```python
from build123d import *

# Parameters (mm, degrees)
SKETCH_R      = 6.05
SKETCH_R_2    = 2.2
PAD_DEPTH     = 6
POCKET_DEPTH  = 3.5
SKETCH002_R   = 8.05
SKETCH002_R_2 = 6.05
PAD001_DEPTH  = 4
CHAMFER_SIZE  = 0.5


with BuildPart() as part:
    # Sketch → Pad (new body)
    with BuildSketch(Plane.XY):
        with BuildLine():
            ThreePointArc((-9.05, 8.05), (-17.1, 0), (-9.05, -8.05))
            Line((-9.05, -8.05), (9.05, -8.05))
            ThreePointArc((9.05, -8.05), (17.1, 0), (9.05, 8.05))
            Line((-9.05, 8.05), (9.05, 8.05))
        make_face()
        Circle(SKETCH_R, mode=Mode.SUBTRACT)
        with Locations((-11.575, 0)):
            Circle(SKETCH_R_2, mode=Mode.SUBTRACT)
        with Locations((11.575, 0)):
            Circle(SKETCH_R_2, mode=Mode.SUBTRACT)
    extrude(amount=PAD_DEPTH)

    # Sketch001 → Pocket (cut)
    with BuildSketch(Plane.XY.offset(6)):
        Polygon((-11.575, -4.070319), (-8.05, -2.03516), (-8.05, 2.03516), (-11.575, 4.070319), (-15.1, 2.03516), (-15.1, -2.03516), align=None)
        Polygon((11.575, -4.070319), (15.1, -2.03516), (15.1, 2.03516), (11.575, 4.070319), (8.05, 2.03516), (8.05, -2.03516), align=None)
    extrude(amount=-POCKET_DEPTH, mode=Mode.SUBTRACT)

    # Sketch002 → Pad001 (new body)
    with BuildSketch(Plane.XY.offset(6)):
        Circle(SKETCH002_R)
        Circle(SKETCH002_R_2, mode=Mode.SUBTRACT)
    extrude(amount=PAD001_DEPTH)

    # Chamfer
    chamfer_edges = [part.edges().sort_by_distance(p)[0] for p in [
        (-13.775, 0, 0),
        (-6.05, 0, 0),
        (9.375, 0, 0),
    ]]
    chamfer(chamfer_edges, length=CHAMFER_SIZE)


solid = part.part
```
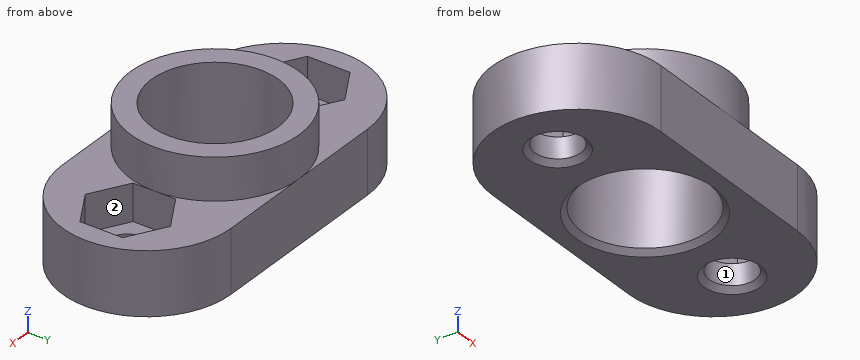
The listing builds one solid part. Answer for the finished solid, in the listing's coordinates (mm). Face numbers are marked on the shaded views. A direction names the side the tool comes from. Give positions to 0.01 mm unless a question says otherwise; leave off trailing zeros. Write each loop counter-clockwise with the first axis right and the second up, starting at its lowest first coordinate (ties: lowest second). Pieces come first, ordered by that corner, then holes. Notation, with made-up numbers: (6, 60.25) - (59, 60.25) arc R9 ccw to (59, 77.25) - close; hole circle Ø8 at (4, -3.5). An arc over 180 degrees is marked (long way). Use one line per item in the form item = value. Start each with the question number.
1) Find section A-A on z = 1.25. Determine the outline of the cut face in (x, y) (3 decimals).
2) Consider line 1 along Y through (x, z) = (0, 6.75); line 2 along X through (y, z) = (3.75, 4.5); line 3 along Z through (x, y) = (10, 6.5). Determine where each line is inside the solid, lowest interval first. Write a range as from..to.
3) Flat-ended cylindrical pins translate along their axes: pin 1 Ø5.5 at (x, y) = (-11.5, -2) entering from +Z; pin 2 Ø5 at (x, y) = (-1.5, 0.5) entering from -Z; pin 3 Ø3.5 at (x, y) = (10.5, -0.5) entering from +Z; pin 4 Ø4 at (y, z) = (-5, 5.5) entering from -X. Find the tip coordinate at first contact, or state that the pin passes through.
4) Find section C-C on y = 0.75. Count the separate pieces of the cut face and the enclosed holes in it, plus the area to 3 significant figures.
5) Find section D-D on z = 7.5. Determine the outline of the cut face in (x, y), plus the area to 3 significant figures.
6) Find section B-B on x = -8.5. Determine the outline of the cut face in (y, z), plus the area to 3 significant figures.
7) A tool of negligible diameter and unlimited length cuts with its end or side. For the marked faces 1 and 2, from which of +Z, -Z, +X, -X, +Y, -Y can it reach the whole face along a straight path? Write none if from no direction.
Geometry results:
q1.outline = (-9.05, -8.05) - (9.05, -8.05) arc R8.05 ccw to (9.05, 8.05) - (-9.05, 8.05) arc R8.05 ccw to start; hole circle Ø4.4 at (-11.575, 0); hole circle Ø12.1 at (0, 0); hole circle Ø4.4 at (11.575, 0)
q2.line_1 = -8.05..-6.05, 6.05..8.05
q2.line_2 = -16.17..-12.13, -11.02..-4.75, 4.75..11.02, 12.13..16.17
q2.line_3 = 0..6
q3.pin_1 = 6
q3.pin_2 = through
q3.pin_3 = 2.5
q3.pin_4 = -16.52
q4.separate_pieces = 4
q4.enclosed_holes = 0
q4.area = 78.0 mm2
q5.outline = circle Ø16.1 at (0, 0); hole circle Ø12.1 at (0, 0)
q5.area = 88.6 mm2
q6.outline = (-8.05, 0) - (8.05, 0) - (8.05, 6) - (2.29, 6) - (2.29, 2.5) - (-2.29, 2.5) - (-2.29, 6) - (-8.05, 6) - close
q6.area = 80.5 mm2
q7.face_1 = +Z, -Z
q7.face_2 = +Z
